Verification items for the finished model (mm, model axes). A direction names the side the tool comes from. Give positions to 0.01 mm unless a question says otherwise; leave off trailing zeros. Order: outer loops, then holes, each group sorted by start corner. A loop starts at its lowest first (then second) coordinate and runs counter-clockwise, first axis right, second up.
(1) Access from +Z, -Z, +X, -X, +Y, -Y to the whole of each face (thin tool, end or side, straight path). Record for faces 1 (the face through (-23.19, 2.01, 4.9)), 2 (the face through (29.075, 11.73, -1.565)).
(2) Scan lines: L1, parallel to X at y = 13.75, z = 0; L2, parallel to X at y = 5.5, z = -0.75; L3, parallel to X at y = 15.25, z = 0. Record each from-to range of solid material in increasing order.
(3) Sectioned sample at D-D on y = 2.25. Record the cut outline in (x, z).
(4) Gauge pin test, flat ends, axial feed: pin 1 (5.5 mm diameter, centred on x = -26.07, z = 0, fed in from -Y); pin 2 (9 mm diameter, centred on x = -25.5, z = 1, fed in from -Y); pin 3 (2 mm diameter, centred on y = 2.5, z = -0.5, fed in from +X). Record the tip position at first contact, or that the pin passes through.
(5) Mould release check, pull along X, two halves, no side actions. Record for faces 3 (the face through (23.485, 18.031, 11.614)), 4 (the face through (35, 1.1, -0.1)), 5 (the face through (-28.95, 2.01, -4.9)), 6 (the face through (-31.75, 2, 0)): pulls with the +X half, pulls with the -X half, needs draft (parallel to the pull), parting line crosses it, or undercut.
(6) Sectioned sample at C-C on x = -17. Record the cut outline in (y, z).
(7) Sectioned sample at B-B on y = 11. Record the cut outline in (x, z).
(8) Sectioned sample at A-A on z = 0. Record the cut outline in (x, y).
```python
from build123d import *

# Parameters (mm, degrees)
BOSS_EXTRUDE1_DEPTH = 12.7
SKETCH2_R           = 3.3909
CUT_EXTRUDE1_DEPTH  = 45.343964598
SKETCH3_W           = 72.263
SKETCH3_H           = 7.175826556
CUT_EXTRUDE2_DEPTH  = 50.500072689
CUT_EXTRUDE3_DEPTH  = 4.07162
FILLET3_R           = 3.81


with BuildPart() as part:
    # Sketch1 → Boss-Extrude1 (new, symmetric)
    with BuildSketch(Plane.XY):
        with BuildLine():
            Line((16.002, 22.352), (36.1315, 22.352))
            Line((36.1315, 22.352), (36.1315, 0))
            Line((36.1315, 0), (-36.1315, 0))
            Line((-36.1315, 0), (-36.1315, 22.352))
            Line((-36.1315, 22.352), (-16.002, 22.352))
            ThreePointArc((-16.002, 22.352), (0, 6.35), (16.002, 22.352))
        make_face()
    extrude(amount=BOSS_EXTRUDE1_DEPTH, both=True)

    # Sketch2 → Cut-Extrude1 (cut, through all)
    with BuildSketch(Plane(origin=(0, 22.352, 0), x_dir=(1, 0, 0), z_dir=(0, 1, 0))):
        with Locations(Location((-26.06675, 0, 0), (0, 0, 270))):
            Circle(SKETCH2_R)
        with Locations(Location((26.06675, 0, 0), (0, 0, 90))):
            Circle(SKETCH2_R)
    extrude(amount=-CUT_EXTRUDE1_DEPTH, mode=Mode.SUBTRACT)

    # Sketch3 → Cut-Extrude2 (cut, through all)
    with BuildSketch(Plane.XY.offset(12.7)):
        with Locations((0, 22.764913278)):
            Rectangle(SKETCH3_W, SKETCH3_H)
    extrude(amount=-CUT_EXTRUDE2_DEPTH, mode=Mode.SUBTRACT)

    # Sketch6 → Cut-Extrude3 (cut)
    with BuildSketch(Plane.XZ):
        Polygon((-26.06675, -6.562451835), (-20.3835, -3.281225917), (-20.3835, 3.281225917), (-26.06675, 6.562451835), (-31.75, 3.281225917), (-31.75, -3.281225917), align=None)
        Polygon((26.06675, 6.562451835), (20.3835, 3.281225917), (20.3835, -3.281225917), (26.06675, -6.562451835), (31.75, -3.281225917), (31.75, 3.281225917), align=None)
    extrude(amount=-CUT_EXTRUDE3_DEPTH, mode=Mode.SUBTRACT)

    # Fillet3
    fillet3_edges = [part.edges().sort_by_distance(p)[0] for p in [
        (36.1315, 9.5885, 12.7),
        (36.1315, 0, 0),
        (-36.1315, 0, 0),
        (-36.1315, 9.5885, -12.7),
        (-36.1315, 9.5885, 12.7),
        (25.907678637, 19.177, 12.7),
        (-25.907678637, 19.177, 12.7),
        (-36.1315, 19.177, 0),
        (-25.907678637, 19.177, -12.7),
        (25.907678637, 19.177, -12.7),
        (36.1315, 19.177, 0),
        (0, 0, 12.7),
        (36.1315, 9.5885, -12.7),
        (0, 0, -12.7),
    ]]
    fillet(fillet3_edges, radius=FILLET3_R)


solid = part.part
```
Ans:
1. face 1: -Y
1. face 2: +Y, -Y
2. L1: x = -36.13 to -29.46, -22.68 to -13.49, 13.49 to 22.68, 29.46 to 36.13
2. L2: x = -36.13 to -29.37, -22.76 to 22.76, 29.37 to 36.13
2. L3: x = -36.13 to -29.46, -22.68 to -14.34, 14.34 to 22.68, 29.46 to 36.13
3. outline: (-35.8, -8.89) arc R3.48 ccw to (-32.32, -12.37) - (32.32, -12.37) arc R3.48 ccw to (35.8, -8.89) - (35.8, 8.89) arc R3.48 ccw to (32.32, 12.37) - (-32.32, 12.37) arc R3.48 ccw to (-35.8, 8.89) - close; hole (-31.75, -3.28) - (-26.07, -6.56) - (-20.38, -3.28) - (-20.38, 3.28) - (-26.07, 6.56) - (-31.75, 3.28) - close; hole (20.38, -3.28) - (26.07, -6.56) - (31.75, -3.28) - (31.75, 3.28) - (26.07, 6.56) - (20.38, 3.28) - close
4. pin 1: passes through
4. pin 2: stops at y = 4.07
4. pin 3: stops at x = 36.12
5. face 3: needs draft
5. face 4: pulls with the +X half
5. face 5: undercut
5. face 6: undercut
6. outline: (0, -8.89) arc R3.81 ccw to (3.81, -12.7) - (15.37, -12.7) arc R3.81 ccw to (19.18, -8.89) - (19.18, 8.89) arc R3.81 ccw to (15.37, 12.7) - (3.81, 12.7) arc R3.81 ccw to (0, 8.89) - close
7. outline: (-36.13, -8.89) arc R3.81 ccw to (-32.32, -12.7) - (-11.28, -12.7) - (-11.28, 12.7) - (-32.32, 12.7) arc R3.81 ccw to (-36.13, 8.89) - close; (11.28, -12.7) - (32.32, -12.7) arc R3.81 ccw to (36.13, -8.89) - (36.13, 8.89) arc R3.81 ccw to (32.32, 12.7) - (11.28, 12.7) - close; hole circle Ø6.78 at (-26.07, 0); hole circle Ø6.78 at (26.07, 0)
8. outline: (-36.13, 3.81) arc R3.81 ccw to (-32.32, 0) - (-31.75, 0) - (-31.75, 4.07) - (-29.46, 4.07) - (-29.46, 19.18) - (-32.32, 19.18) arc R3.81 ccw to (-36.13, 15.37) - close; (-22.68, 4.07) - (-20.38, 4.07) - (-20.38, 0) - (20.38, 0) - (20.38, 4.07) - (22.68, 4.07) - (22.68, 19.18) - (15.68, 19.18) arc R16 cw to (-15.68, 19.18) - (-22.68, 19.18) - close; (29.46, 4.07) - (31.75, 4.07) - (31.75, 0) - (32.32, 0) arc R3.81 ccw to (36.13, 3.81) - (36.13, 15.37) arc R3.81 ccw to (32.32, 19.18) - (29.46, 19.18) - close
